from build123d import *

# Parameters (mm, degrees)
F0_R     = 47.625
F0_R_2   = 5.55625
F1_DEPTH = 3.048


with BuildPart() as f1:
    # F0 (on Right) → F1 (new body)
    with BuildSketch(Plane.YZ):
        Circle(F0_R)
        with Locations((-26.9407683632, -26.9407683632)):
            Circle(F0_R_2, mode=Mode.SUBTRACT)
        with Locations((26.9407683632, -26.9407683632)):
            Circle(F0_R_2, mode=Mode.SUBTRACT)
        with Locations((-26.9407683632, 26.9407683632)):
            Circle(F0_R_2, mode=Mode.SUBTRACT)
        with BuildLine():
            ThreePointArc((11.176, 24.4948729329), (0, -26.924), (-11.176, 24.4948729329))
            Line((-11.176, 24.4948729329), (-11.176, 33.274))
            Line((-11.176, 33.274), (11.176, 33.274))
            Line((11.176, 33.274), (11.176, 24.4948729329))
        make_face(mode=Mode.SUBTRACT)
        with Locations((26.9407683632, 26.9407683632)):
            Circle(F0_R_2, mode=Mode.SUBTRACT)
    extrude(amount=F1_DEPTH)


solid = f1.part
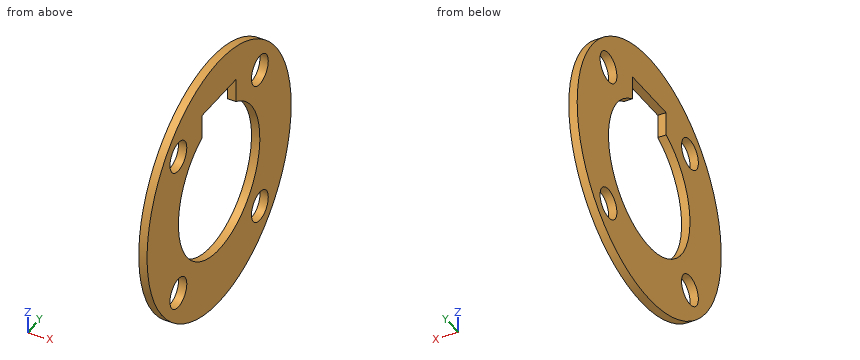
Geometry: final body of the model. Coordinates: model frame, mm. Round coordinates to 2 decimals unless told otherwise and drop trailing zeros. Loops run counter-clockwise (first coordinate to the right, second up) from the corner with the lowest first, then second, coordinate; pieces in that order, holes last.
Q1. Section D-D on y = 25. Return loops of the section in (x, z), plus the area to 3 significant figures.
Q2. Material intervals for L1, parallel to Z at x = 2.45, y = 29.5; L2, parallel to Y at x = 1.15, z = -27; L3, parallel to Z at x = 2, y = 0 (3 decimals), sorted ascending.
Q3. Pin query (flat end, axial travel): P1, Ø0.9, axis at x = 1, z = 28.5, coming from the +Y side; P2, Ø1.5, axis at x = 2.5, y = -26, coming from the +Z side; P3, Ø0.9, axis at x = 1, y = 5, coming from the -Z side; P4, Ø9, axis at y = 26.94, z = 26.94, coming from the +X side. Return the tip coordinate at first contact, or that it passes through.
Q4. Section A-A on y = 0. Return loops of the section in (x, z) (3 decimals), plus the area to 3 significant figures.
Q5. Section C-C on x = 1.75. State how many separate pieces and enclosed holes the cut face has, plus the area to 3 significant figures.
Q6. Section B-B on z = 0. Return loops of the section in (x, y) (3 decimals).
Evaluation:
1. outline: (0, -40.54) - (3.05, -40.54) - (3.05, -32.15) - (0, -32.15) - close; (0, -21.73) - (3.05, -21.73) - (3.05, -10) - (0, -10) - close; (0, 10) - (3.05, 10) - (3.05, 21.73) - (0, 21.73) - close; (0, 32.15) - (3.05, 32.15) - (3.05, 40.54) - (0, 40.54) - close
1. area: 123 mm2
2. L1: z = -37.39 to -31.87, -22.01 to 22.01, 31.87 to 37.39
2. L2: y = -39.23 to -32.5, -21.38 to 21.38, 32.5 to 39.23
2. L3: z = -47.625 to -26.924, 33.274 to 47.625
3. P1: stops at y = 38.49
3. P2: stops at z = 40.38
3. P3: stops at z = -47.41
3. P4: passes through
4. outline: (0, -47.625) - (3.048, -47.625) - (3.048, -26.924) - (0, -26.924) - close; (0, 33.274) - (3.048, 33.274) - (3.048, 47.625) - (0, 47.625) - close
4. area: 107 mm2
5. separate pieces: 1
5. enclosed holes: 5
5. area: 4,300 mm2
6. outline: (0, -47.625) - (3.048, -47.625) - (3.048, -26.924) - (0, -26.924) - close; (0, 26.924) - (3.048, 26.924) - (3.048, 47.625) - (0, 47.625) - close
